Autodesk Inventor part; units mm, degrees
ref_plane "YZ Plane" through (0, 0, 0) normal (1, 0, 0) x (0, 1, 0)
ref_plane "XZ Plane" through (0, 0, 0) normal (0, 1, 0) x (-1, 0, 0)
ref_plane "XY Plane" through (0, 0, 0) normal (0, 0, 1) x (1, 0, 0)
sketch "Sketch1" plane through (0, 0, 0) normal (0, 1, 0) x (-1, 0, 0)
  line L0 (0, 0) -> (-50, 0)
  line L1 (-50, 0) -> (-50, -23)
  line L2 (-50, -23) -> (0, -23)
  line L3 (0, -23) -> (0, 0)
  dimension "d0" = 50
  dimension "d1" = 23
extrude "Extrusion1" add sketch "Sketch1" along normal blind 3
sketch "Sketch2" plane through (0, 3, 0) normal (0, 1, 0) x (1, 0, 0)
  line L0 (0, 23) -> (0, 0) construction
  line L1 (0, 0) -> (50, 0) construction
  line L2 (50, 0) -> (50, 23) construction
  line L3 (0, 3) -> (50, 3)
  line L4 (50, 3) -> (50, 0)
  line L5 (50, 0) -> (0, 0)
  line L6 (0, 0) -> (0, 3)
  dimension "d4" = 3
extrude "Extrusion2" add sketch "Sketch2" along normal blind 20
sketch "Sketch3" plane through (0, 0, 0) normal (0, 0, 1) x (1, 0, 0)
  circle A0 centre (6.5, 13) radius 1.6
  circle A1 centre (43.5, 13) radius 1.6
  line L0 (0, 0) -> (0, 23)
  line L1 (0, 23) -> (50, 23)
  dimension "d7" = 3.2
  dimension "d8" = 3.2
  dimension "d9" = 37
  dimension "d10" = 6.5
  dimension "d11" = 10
  dimension "d12" = 10
extrude "Extrusion3" cut sketch "Sketch3" against normal through all
fillet "Fillet1" radius 6 4 edges at (0, 23, -1.5) (50, 23, -1.5) (0, 1.5, -23) (50, 1.5, -23)
sketch "Sketch4" plane through (0, 3, 0) normal (0, 1, 0) x (1, 0, 0)
  circle A0 centre (35, 13) radius 1.6
  circle A1 centre (15, 13) radius 1.6
  line L0 (44, 23) -> (6, 23)
  line L1 (50, 3) -> (50, 17)
  point P0 (0, 0)
  point P1 (50, 5)
  dimension "d17" = 3.2
  dimension "d18" = 3.2
  dimension "d19" = 10
  dimension "d20" = 20
  dimension "d21" = 15
extrude "Extrusion4" cut sketch "Sketch4" against normal through all
equation "\"d8\" = d7"
equation "\"d12\" = d11"
properties part number "FrontIRHolder"
Build history of the part. All positions in model axes, mm. A direction names the side the tool comes from. Give positions to 0.01 mm unless a question says otherwise; leave off trailing zeros. Order: outer loops, then holes, each group sorted by start corner. A loop starts at its lowest first (then second) coordinate and runs counter-clockwise, first axis right, second up. Notation, with made-up numbers: M 71.5,-6.5 L 79.5,-6.5 A24 cw 79.5,15.5 Z; hole C 46.5,-21.75 d1. An arc over 180 degrees is marked long. Use one line per item in the form item = value.
Q1. Which spindle directions (+Z, -Z, +X, -X, +Y, -Y) get a long thin tool onto all of the face, cutting with end or side? Do faces 4 (the flat face through (25, 3, -13)), 5 (the cylindrical face through (43.292, 14.586, -1.479)). Say none if no direction does.
Conclusion:
face_4 = -Z, +X, -X, +Y
face_5 = +Z, -Z
Q2. Slice it at A-A, the plane y = 13. Write the cut outline in (x, z).
Conclusion:
outline = M 0,-3 L 4.9,-3 L 4.9,0 L 0,0 Z; M 8.1,-3 L 41.9,-3 L 41.9,0 L 8.1,0 Z; M 45.1,-3 L 50,-3 L 50,0 L 45.1,0 Z
Q3. Pin check, flat tips, straight feed: P1, Ø6, axis at x = 29, z = -20, coming from the +Y side; P2, Ø4, axis at x = 43.5, y = 13, coming from the -Z side; P3, Ø2, axis at x = 27.5, z = -6.5, coming from the -Y side. Stop position of each tip, or through.
Conclusion:
P1 = 3
P2 = -3
P3 = 0
Q4. Slice it at D-D, the plane x = 28. Write the cut outline in (y, z).
Conclusion:
outline = M 0,-23 L 3,-23 L 3,-3 L 23,-3 L 23,0 L 0,0 Z
Q5. Slice it at B-B, the plane z = -13. Write the cut outline in (x, y).
Conclusion:
outline = M 0,0 L 13.4,0 L 13.4,3 L 0,3 Z; M 16.6,0 L 33.4,0 L 33.4,3 L 16.6,3 Z; M 36.6,0 L 50,0 L 50,3 L 36.6,3 Z
Q6. Wall check: probe 1 along X at (y, z) = (1.9, -13); probe 2 along Z at (x, y) = (15, 1.9); probe 3 along Y at (x, z) = (12, -7). Give the ranges that are in metal, low to high.
Conclusion:
probe_1 = 0 to 13.4, 16.6 to 33.4, 36.6 to 50
probe_2 = -23 to -14.6, -11.4 to 0
probe_3 = 0 to 3
Q7. Slice it at C-C, the plane x = 6.5. Write the cut outline in (y, z).
Conclusion:
outline = M 0,-23 L 3,-23 L 3,-3 L 11.4,-3 L 11.4,0 L 0,0 Z; M 14.6,-3 L 23,-3 L 23,0 L 14.6,0 Z
Q8. Pull direction X, two halves, no side cores. Call faces 1 (the cylindrical face through (33.82, 1.52, -14.08)), 2 (the cylindrical face through (1.711, 21.196, -1.521)), 3 (the flat face through (25, 23, -2)): released by +X, released by -X, zero draft, split by the parting line, or undercut.
Conclusion:
face_1 = undercut
face_2 = released by -X
face_3 = zero draft
